Check sheet for the modelled part. Datum: model origin and axes. Units: mm. A direction names the side the tool comes from. Round coordinates to 2 decimals unless told otherwise and drop trailing zeros. Write each loop counter-clockwise with the first axis right and the second up, starting at its lowest first coordinate (ties: lowest second). Pieces come first, ordered by that corner, then holes. Notation, with made-up numbers: (23.25, 41) -> (54.25, 41) arc R3 cw to (54.25, 46) -> close; hole circle Ø9 at (-33, 7.25). An arc over 180 degrees is marked (long way). Write item = value, one per line.
from build123d import *

# Parameters (mm, degrees)
F0_R     = 18.5
F1_DEPTH = 50
F0_R_2   = 16.5
F2_DEPTH = 25
F3_R     = 2.5
F4_DEPTH = 35
F3_R_2   = 4
F5_DEPTH = 21


with BuildPart() as f1:
    # F0 (on Top) → F1 (new body)
    with BuildSketch(Plane.XY):
        with BuildLine():
            ThreePointArc((18.484245, 10.981015), (20.732357, 5.693801), (21.5, 0))
            ThreePointArc((21.5, 0), (-5.693801, -20.732357), (-18.484245, 10.981015))
            Line((-18.484245, 10.981015), (-41.20501, -27.264646))
            ThreePointArc((-41.20501, -27.264646), (-41.223789, -29.275332), (-39.485546, -30.286135))
            Line((-39.485546, -30.286135), (0, -30.286135))
            Line((0, -30.286135), (39.485546, -30.286135))
            ThreePointArc((39.485546, -30.286135), (41.223789, -29.275332), (41.20501, -27.264646))
            Line((41.20501, -27.264646), (18.484245, 10.981015))
        make_face()
        with BuildLine():
            ThreePointArc((-18.484245, 10.981015), (-5.693801, -20.732357), (21.5, 0))
            ThreePointArc((21.5, 0), (20.732357, 5.693801), (18.484245, 10.981015))
            ThreePointArc((18.484245, 10.981015), (0, 21.5), (-18.484245, 10.981015))
        make_face()
        Circle(F0_R, mode=Mode.SUBTRACT)
    extrude(amount=F1_DEPTH)

    # F0 (on Top) → F2 (join)
    with BuildSketch(Plane.XY):
        Circle(F0_R)
        Circle(F0_R_2, mode=Mode.SUBTRACT)
    extrude(amount=F2_DEPTH)

    # F3 (on Front) → F4 (cut)
    with BuildSketch(Plane.XZ):
        with Locations((33, 24.184783)):
            Circle(F3_R)
        with Locations((-33, 24.184783)):
            Circle(F3_R)
    extrude(amount=F4_DEPTH, mode=Mode.SUBTRACT)

    # F3 (on Front) → F5 (cut)
    with BuildSketch(Plane.XZ):
        with Locations((33, 24.184783)):
            Circle(F3_R_2)
        with Locations((33, 24.184783)):
            Circle(F3_R, mode=Mode.SUBTRACT)
        with Locations((-33, 24.184783)):
            Circle(F3_R_2)
        with Locations((-33, 24.184783)):
            Circle(F3_R, mode=Mode.SUBTRACT)
    extrude(amount=F5_DEPTH, mode=Mode.SUBTRACT)


solid = f1.part
(1) Sectioned sample at D-D on z = 35. Enter the section's corners in (x, y).
Worked answers:
outline = (-41.21, -27.26) arc R2 ccw to (-39.49, -30.29) -> (39.49, -30.29) arc R2 ccw to (41.21, -27.26) -> (18.48, 10.98) arc R21.5 ccw to (-18.48, 10.98) -> close; hole circle Ø37 at (0, 0)
(2) Sectioned sample at A-A on z = 16. Enter the section's corners in (x, y), then the cut area to 3 significant figures.
Worked answers:
outline = (-41.21, -27.26) arc R2 ccw to (-39.49, -30.29) -> (39.49, -30.29) arc R2 ccw to (41.21, -27.26) -> (18.48, 10.98) arc R21.5 ccw to (-18.48, 10.98) -> close; hole circle Ø33 at (0, 0)
area = 1,950 mm²
(3) Sectioned sample at C-C on y = 0. Enter the section's corners in (x, z).
Worked answers:
outline = (-25.01, 0) -> (-16.5, 0) -> (-16.5, 25) -> (-18.5, 25) -> (-18.5, 50) -> (-25.01, 50) -> close; (16.5, 0) -> (25.01, 0) -> (25.01, 50) -> (18.5, 50) -> (18.5, 25) -> (16.5, 25) -> close
(4) Release check for a two-part mould opening along Y. For faces 1 (the cylindrical face through (15.24, -6.32, 12.32)), 2 (the flat face through (-17, 0, 25)), 3 (the cylindrical face through (0.311, 21.498, 24.65)), 4 (the cylindrical face through (32.675, -25.578, 26.664)) record: pulls with the +Y half, pulls with the -Y half, needs draft (parallel to the pull), parting line crosses it, or undercut.
Worked answers:
face_1 = undercut
face_2 = undercut
face_3 = pulls with the +Y half
face_4 = needs draft
(5) Sectioned sample at B-B on x = 0. Enter the section's corners in (y, z), then the cut area to 3 significant figures.
Worked answers:
outline = (-30.29, 0) -> (-16.5, 0) -> (-16.5, 25) -> (-18.5, 25) -> (-18.5, 50) -> (-30.29, 50) -> close; (16.5, 0) -> (21.5, 0) -> (21.5, 50) -> (18.5, 50) -> (18.5, 25) -> (16.5, 25) -> close
area = 839 mm²
(6) Access from +Z, -Z, +X, -X, +Y, -Y to the whole of each face (thin tool, end or side, straight path). Record for faces 5 (the cylindrical face through (-4.01, -18.06, 37.33)), 6 (the flat face through (35, -21, 26)), 7 (the flat face through (-27.16, -3.62, 24.65)).
Worked answers:
face_5 = +Z
face_6 = +Y
face_7 = +Z, -Z, -X, +Y
(7) Material ranges on L1, parallel to Y at x = 0, z = 14.75; L2, parallel to Y at x = 0, z = 30.5; L3, parallel to Z at x = -33, y = -23, recorded low to high. Write a range as [from, to].
Worked answers:
L1 = [-30.29, -16.5], [16.5, 21.5]
L2 = [-30.29, -18.5], [18.5, 21.5]
L3 = [0, 21.68], [26.68, 50]
(8) Go/stop test with flat-tipped pins: P1, Ø1, axis at x = 0, z = 44, coming from the +Y side; P2, Ø5, axis at x = -8, z = 16, coming from the +Y side; P3, Ø9, axis at x = -33.5, z = 23, coming from the +Y side; P4, Ø11, axis at x = -6, y = -3, coming from the +Z side. Record where each tip stops, or that it passes through.
Worked answers:
P1 = 21.5
P2 = 20.78
P3 = -6.72
P4 = through
